Geometry: final body of the model. Coordinates: model frame, mm. Give positions to 0.01 mm unless a question says otherwise; leave off trailing zeros. Loops run counter-clockwise (first coordinate to the right, second up) from the corner with the lowest first, then second, coordinate; pieces in that order, holes last. Notation, with made-up numbers: (-10, -28.75) -> (-1, -28.75) arc R22 ccw to (-1, -3.75) -> close; hole circle Ø4 at (-0.75, 76). An arc over 180 degrees is marked (long way). Answer in a Markdown table with one row per item. Add a question column.
1) First-contact query: P1, Ø1, axis at x = 139.5, z = 2, coming from the -Y side; P2, Ø1.6, axis at y = 23, z = 1.5, coming from the +X side; P3, Ø1.6, axis at x = 164, z = 1.5, coming from the +Y side; P4, Ø2, axis at x = -7.75, y = 23.98, coming from the -Z side. Flat tips, straight axial feed; report the tip coordinate or a pass-through.
2) Line query: line 1 (X direction, y = 18, z = 0.1); line 2 (X direction, y = -1, z = 1); line 3 (Y direction, x = -18, z = 1.15). Output: solid intervals per line, ascending. Write a range as from..to.
3) Section query B-B (x = 32.5). Return the cut outline in (y, z) (3 decimals).
4) Section query C-C (z = 2.5). Give the number of separate pieces and of enclosed holes in the cut face, plus the area to 3 significant figures.
5) Section query A-A (y = -56.5). Return the cut outline in (x, z) (3 decimals), plus the area to 3 significant figures.
```python
from build123d import *

# Parameters (mm, degrees)
SKETCH1_W               = 215.9
SKETCH1_H               = 127
BOSS_EXTRUDE1_DEPTH     = 3.175
SKETCH4_W               = 11.35
SKETCH4_H               = 13.0800094
SKETCH4_W_2             = 101.949970282
SKETCH4_W_3             = 11.50001
SKETCH4_W_4             = 102.400000282
CUT_EXTRUDE1_DEPTH      = 4.175
SKETCH5_R               = 6
CUT_EXTRUDE2_DEPTH      = 1
CUT_EXTRUDE2_DEPTH_BACK = 4.175
SKETCH6_R               = 1.7145
CUT_EXTRUDE3_DEPTH      = 4.175
SKETCH10_W              = 3.175
SKETCH10_H              = 11.34999
CUT_EXTRUDE4_DEPTH      = 3.175


with BuildPart() as part:
    # Sketch1 → Boss-Extrude1 (new body)
    with BuildSketch(Plane.XY):
        with Locations((60.172222222, -34.055555556)):
            Rectangle(SKETCH1_W, SKETCH1_H)
    extrude(amount=BOSS_EXTRUDE1_DEPTH)

    # Sketch4 → Cut-Extrude1 (cut, through all)
    with BuildSketch(Plane(origin=(0, 0, 0), x_dir=(-1, 0, 0), z_dir=(0, 0, -1))):
        with Locations((-162.447222222, 22.904439744)):
            Rectangle(SKETCH4_W, SKETCH4_H)
        with Locations((-139.747222222, 22.904439744)):
            Rectangle(SKETCH4_W, SKETCH4_H)
        with Locations((-71.747237175, 22.904439744)):
            Rectangle(SKETCH4_W_2, SKETCH4_H)
        with Locations((-3.672247128, 22.904439744)):
            Rectangle(SKETCH4_W_3, SKETCH4_H)
        with Locations((19.177762872, 22.904439744)):
            Rectangle(SKETCH4_W_3, SKETCH4_H)
        with Locations((42.027772778, 22.904439744)):
            Rectangle(SKETCH4_W_3, SKETCH4_H)
        with Locations((-162.447222222, -91.015550856)):
            Rectangle(SKETCH4_W, SKETCH4_H)
        with Locations((-139.747222222, -91.015550856)):
            Rectangle(SKETCH4_W, SKETCH4_H)
        with Locations((-71.522222175, -91.015550856)):
            Rectangle(SKETCH4_W_4, SKETCH4_H)
        with Locations((-3.297222034, -91.015550856)):
            Rectangle(SKETCH4_W, SKETCH4_H)
        with Locations((19.402777872, -91.015550856)):
            Rectangle(SKETCH4_W, SKETCH4_H)
        with Locations((42.102777778, -91.015550856)):
            Rectangle(SKETCH4_W, SKETCH4_H)
    extrude(amount=-CUT_EXTRUDE1_DEPTH, mode=Mode.SUBTRACT)

    # Sketch5 → Cut-Extrude2 (cut, two sides)
    with BuildSketch(Plane(origin=(0, 0, 0), x_dir=(-1, 0, 0), z_dir=(0, 0, -1))) as cut_extrude2_sk:
        with Locations((-138.137522222, -65.425546156)):
            Circle(SKETCH5_R)
        with Locations((17.793077778, -65.425546156)):
            Circle(SKETCH5_R)
    extrude(amount=CUT_EXTRUDE2_DEPTH, mode=Mode.SUBTRACT)
    extrude(cut_extrude2_sk.sketch, amount=-CUT_EXTRUDE2_DEPTH_BACK, mode=Mode.SUBTRACT)

    # Sketch6 → Cut-Extrude3 (cut, through all)
    with BuildSketch(Plane(origin=(0, 0, 0), x_dir=(-1, 0, 0), z_dir=(0, 0, -1))):
        with Locations((-151.097222222, 23.984435044)):
            Circle(SKETCH6_R)
        with Locations((-128.397222269, 23.984435044)):
            Circle(SKETCH6_R)
        with Locations((-15.097252081, 23.984435044)):
            Circle(SKETCH6_R)
        with Locations((7.752757872, 23.984435044)):
            Circle(SKETCH6_R)
        with Locations((30.602767825, 23.984435044)):
            Circle(SKETCH6_R)
        with Locations((-128.397222269, -92.095546156)):
            Circle(SKETCH6_R)
        with Locations((-151.097222222, -92.095546156)):
            Circle(SKETCH6_R)
        with Locations((-14.647222034, -92.095546156)):
            Circle(SKETCH6_R)
        with Locations((8.052777919, -92.095546156)):
            Circle(SKETCH6_R)
        with Locations((30.752777825, -92.095546156)):
            Circle(SKETCH6_R)
    extrude(amount=-CUT_EXTRUDE3_DEPTH, mode=Mode.SUBTRACT)

    # Sketch10 → Cut-Extrude4 (cut)
    with BuildSketch(Plane.XY.offset(3.175)):
        with Locations((-39.840277778, -1.410561156)):
            Rectangle(SKETCH10_W, SKETCH10_H)
        with Locations((-39.840277778, -53.400551156)):
            Rectangle(SKETCH10_W, SKETCH10_H)
        with Locations((160.184722222, -1.410561156)):
            Rectangle(SKETCH10_W, SKETCH10_H)
        with Locations((160.184722222, -53.400551156)):
            Rectangle(SKETCH10_W, SKETCH10_H)
    extrude(amount=-CUT_EXTRUDE4_DEPTH, mode=Mode.SUBTRACT)


solid = part.part
```
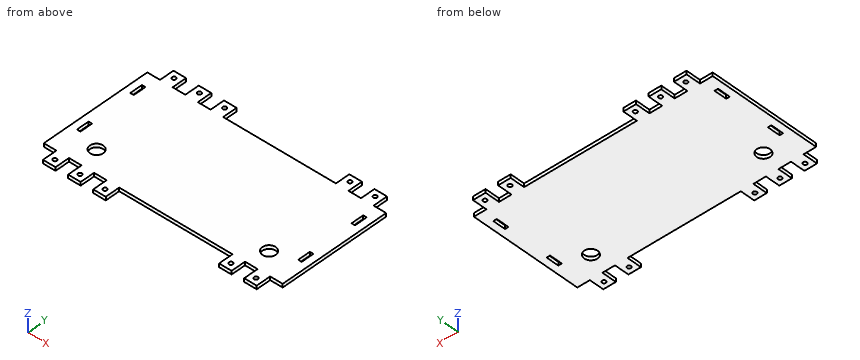
Evaluation:
| question | item | result |
|---|---|---|
| 1 | P1 | y = -84.48 |
| 1 | P2 | x = 156.77 |
| 1 | P3 | y = 16.36 |
| 1 | P4 | through |
| 2 | line 1 | -36.28..-24.93, -13.43..-2.08, 9.42..20.77, 122.72..134.07, 145.42..156.77 |
| 2 | line 2 | -47.78..-41.43, -38.25..158.6, 161.77..168.12 |
| 2 | line 3 | -84.48..-71.42, -59.43..16.36 |
| 3 | outline | (-84.476, 0) -> (16.364, 0) -> (16.364, 3.175) -> (-84.476, 3.175) -> close |
| 4 | separate pieces | 1 |
| 4 | enclosed holes | 16 |
| 4 | area | 22,800 mm² |
| 5 | outline | (-47.778, 0) -> (-41.428, 0) -> (-41.428, 3.175) -> (-47.778, 3.175) -> close; (-38.253, 0) -> (158.597, 0) -> (158.597, 3.175) -> (-38.253, 3.175) -> close; (161.772, 0) -> (168.122, 0) -> (168.122, 3.175) -> (161.772, 3.175) -> close |
| 5 | area | 665 mm² |
